```python
from build123d import *

# Parameters (mm, degrees)
SKETCH2_W           = 70
SKETCH2_H           = 70
BOSS_EXTRUDE1_DEPTH = 8
SKETCH4_W           = 70
SKETCH4_H           = 8
BOSS_EXTRUDE2_DEPTH = 65
SKETCH6_R           = 1.75
CUT_EXTRUDE1_DEPTH  = 10
SKETCH7_R           = 3.5
CUT_EXTRUDE2_DEPTH  = 3
SKETCH9_W           = 21
SKETCH9_H           = 40.5
CUT_EXTRUDE3_DEPTH  = 10
SKETCH10_R          = 2.25
CUT_EXTRUDE4_DEPTH  = 10
FILLET1_R           = 15
FILLET2_R           = 15


with BuildPart() as part:
    # Sketch2 → Boss-Extrude1 (new body)
    with BuildSketch(Plane(origin=(0, 0, 0), x_dir=(1, 0, 0), z_dir=(0, 1, 0))):
        with Locations((20, 2.5)):
            Rectangle(SKETCH2_W, SKETCH2_H)
    extrude(amount=BOSS_EXTRUDE1_DEPTH)

    # Sketch4 → Boss-Extrude2 (add)
    with BuildSketch(Plane(origin=(0, 0, 0), x_dir=(-1, 0, 0), z_dir=(0, -1, 0))):
        with Locations((-20, -28.5)):
            Rectangle(SKETCH4_W, SKETCH4_H)
    extrude(amount=BOSS_EXTRUDE2_DEPTH)

    # Sketch6 → Cut-Extrude1 (cut)
    with BuildSketch(Plane(origin=(0, 0, 24.5), x_dir=(-1, 0, 0), z_dir=(0, 0, -1))):
        with Locations((-50, -7)):
            Circle(SKETCH6_R)
        with Locations((0, -7)):
            Circle(SKETCH6_R)
        with Locations((-50, -57)):
            Circle(SKETCH6_R)
        with Locations((0, -57)):
            Circle(SKETCH6_R)
    extrude(amount=-CUT_EXTRUDE1_DEPTH, mode=Mode.SUBTRACT)

    # Sketch7 → Cut-Extrude2 (cut)
    with BuildSketch(Plane(origin=(0, 0, 24.5), x_dir=(-1, 0, 0), z_dir=(0, 0, -1))):
        with Locations((-50, -7)):
            Circle(SKETCH7_R)
        with Locations((0, -7)):
            Circle(SKETCH7_R)
        with Locations((0, -57)):
            Circle(SKETCH7_R)
        with Locations((-50, -57)):
            Circle(SKETCH7_R)
    extrude(amount=-CUT_EXTRUDE2_DEPTH, mode=Mode.SUBTRACT)

    # Sketch9 → Cut-Extrude3 (cut)
    with BuildSketch(Plane(origin=(0, 8, 0), x_dir=(1, 0, 0), z_dir=(0, 1, 0))):
        with Locations((0.25, 2.25)):
            Rectangle(SKETCH9_W, SKETCH9_H)
    extrude(amount=-CUT_EXTRUDE3_DEPTH, mode=Mode.SUBTRACT)

    # Sketch10 → Cut-Extrude4 (cut)
    with BuildSketch(Plane(origin=(0, 8, 0), x_dir=(1, 0, 0), z_dir=(0, 1, 0))):
        with Locations(Location((-5, 27, 0), (0, 0, 270))):
            Circle(SKETCH10_R)
        with Locations(Location((5, 27, 0), (0, 0, 270))):
            Circle(SKETCH10_R)
        with Locations(Location((-5, -22.5, 0), (0, 0, 270))):
            Circle(SKETCH10_R)
        with Locations(Location((5, -22.5, 0), (0, 0, 270))):
            Circle(SKETCH10_R)
    extrude(amount=-CUT_EXTRUDE4_DEPTH, mode=Mode.SUBTRACT)

    # Fillet1
    fillet1_edges = [part.edges().sort_by_distance(p)[0] for p in [
        (55, 4, -37.5),
    ]]
    fillet(fillet1_edges, radius=FILLET1_R)

    # Fillet2
    fillet2_edges = [part.edges().sort_by_distance(p)[0] for p in [
        (-15, 4, -37.5),
    ]]
    fillet(fillet2_edges, radius=FILLET2_R)


solid = part.part
```
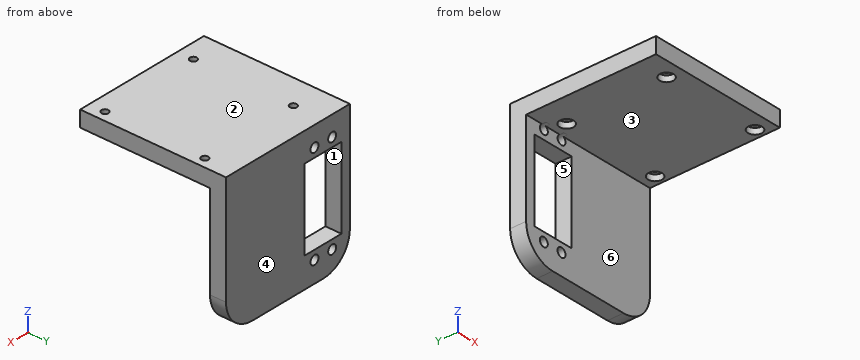
Check sheet for the modelled part. Datum: model origin and axes. Units: mm. Face numbers are marked on the shaded views. A direction names the side the tool comes from. Give positions to 0.01 mm unless a question says otherwise; leave off trailing zeros. Write each loop counter-clockwise with the first axis right and the second up, starting at its lowest first coordinate (ties: lowest second). Pieces come first, ordered by that corner, then holes.
Item 1: Cross-section at D-D (x = 13.5). Enter the section's corners in (y, z).
Item 2: Cross-section at C-C (y = -7). Enter the section's corners in (x, z), and give its area (3 significant figures).
Item 3: Scan lines: L1, parallel to Y at x = 50, z = 31.35; L2, parallel to X at y = 5, z = 7.5; L3, parallel to X at y = 3, z = -27. Record each from-to range of solid material in increasing order.
Item 4: Draft check along Z on the marked faces 1, 2 and 3. Enter one of: released by +Z, released by -Z, zero draft, split by the parting line, or undercut.
Item 5: Access from +Z, -Z, +X, -X, +Y, -Y to the whole of each face (thin tool, end or side, straight path). Record for the marked faces 4, 5 and 6.
Item 6: Gauge pin test, flat ends, axial feed: pin 1 (19.5 mm diameter, centred on x = 8.5, y = -24.5, fed in from -Z); pin 2 (6 mm diameter, centred on x = 9.5, z = -25, fed in from -Y). Record the tip position at first contact, or that the pin passes through.
Item 7: Cross-section at A-A (z = -5). Enter the section's corners in (x, y).
Item 8: Cross-section at B-B (z = 22.5). Enter the section's corners in (x, y), and give its area (3 significant figures).
Report:
1. outline: (-65, 24.5) - (0, 24.5) - (0, -37.5) - (8, -37.5) - (8, 32.5) - (-65, 32.5) - close
2. outline: (-15, 24.5) - (-3.5, 24.5) - (-3.5, 27.5) - (-1.75, 27.5) - (-1.75, 32.5) - (-15, 32.5) - close; (1.75, 27.5) - (3.5, 27.5) - (3.5, 24.5) - (46.5, 24.5) - (46.5, 27.5) - (48.25, 27.5) - (48.25, 32.5) - (1.75, 32.5) - close; (51.75, 27.5) - (53.5, 27.5) - (53.5, 24.5) - (55, 24.5) - (55, 32.5) - (51.75, 32.5) - close
2. area: 483 mm2
3. L1: y = -65 to -58.75, -55.25 to -8.75, -5.25 to 8
3. L2: x = -15 to -10.25, 10.75 to 55
3. L3: x = -14.31 to -7.25, -2.75 to 2.75, 7.25 to 54.31
4. face 1: undercut
4. face 2: released by +Z
4. face 3: released by -Z
5. face 4: +Z, -Z, +X, -X, +Y
5. face 5: +Y, -Y
5. face 6: -Z, +X, -X, -Y
6. pin 1: stops at z = 24.5
6. pin 2: stops at y = 0
7. outline: (-15, 0) - (-10.25, 0) - (-10.25, 8) - (-15, 8) - close; (10.75, 0) - (55, 0) - (55, 8) - (10.75, 8) - close
8. outline: (-15, 0) - (-7.25, 0) - (-7.25, 8) - (-15, 8) - close; (-2.75, 0) - (2.75, 0) - (2.75, 8) - (-2.75, 8) - close; (7.25, 0) - (55, 0) - (55, 8) - (7.25, 8) - close
8. area: 488 mm2
